Geometry check sheet. Reference: the model listing, model coordinates, mm. A direction names the side the tool comes from. Give positions to 0.01 mm unless a question says otherwise; leave off trailing zeros. Write each loop counter-clockwise with the first axis right and the second up, starting at its lowest first coordinate (ties: lowest second). Pieces come first, ordered by that corner, then holes. Notation, with made-up numbers: (-24, 79) -> (1, 79) arc R36 ccw to (1, 113) -> close; hole circle Ø2 at (58, -24.75). An arc over 180 degrees is marked (long way). Write item = value, one per line. Start each with the question number.
1. Depth check by flat-ended pin: P1, Ø4, axis at y = 3, z = -47, coming from the +X side; P2, Ø1, axis at x = -15.5, z = 21.5, coming from the -Y side; P3, Ø12, axis at x = 24, z = 34, coming from the +Y side. Enter the tip coordinate at first touch or a pass-through.
2. Cross-section at B-B, the plane x = -3.5. Record the cut outline in (y, z).
3. Mould release check, pull along X, two halves, no side actions. Record for faces 1 (the flat face through (34, -23.2, -20.9)), 2 (the cylindrical face through (-90.93, 39.923, -20.765)), 3 (the flat face through (10, -29, -70)): pulls with the +X half, pulls with the -X half, needs draft (parallel to the pull), parting line crosses it, or undercut.
4. Thickness scan on line 1 along Y through (x, z) = (37.7, 0); line 2 along Y through (x, z) = (35.45, 0); line 3 along X through (y, z) = (-13, -29). Record the ranges inside material, lowest first.
5. Set-up check for faces 4 (the flat face through (37.5, -12, -29)), 5 (the flat face through (-150, 1, -1)), 6 (the flat face through (47, 0, 0)), 7 (the cylindrical face through (-122.62, 37.18, -4.88)): record each of +Z, -Z, +X, -X, +Y, -Y from which the full face is reachable in a straight line by a thin tool's end or side.
6. Cross-section at A-A, the plane x = -120. Record the cut outline in (y, z), plus the area to 3 significant figures.
```python
from build123d import *

# Parameters (mm, degrees)
FILLET_1_R      = 5
FILLET_2_R      = 10
SKETCH_2_R      = 45
SKETCH_2_R_2    = 35
EXTRUDE_1_DEPTH = 32
SKETCH_3_R      = 35
EXTRUDE_2_DEPTH = 66
SKETCH_4_R      = 37.5
EXTRUDE_3_DEPTH = 54
SKETCH_5_R      = 45
EXTRUDE_4_DEPTH = 10
SKETCH_6_R      = 37.5
EXTRUDE_5_DEPTH = 54
SKETCH_9_R      = 31
EXTRUDE_8_DEPTH = 3.5
SKETCH_10_R     = 32.5
EXTRUDE_9_DEPTH = 9.5


with BuildPart() as part:
    # Sketch 1 → Revolve 1 (revolve)
    with BuildSketch(Plane.XY, mode=Mode.PRIVATE) as revolve_1_sk:
        Polygon((10, 100), (50, 100), (50, 55), (40, 55), (40, 35), (0, 35), (0, 70), (10, 70), align=None)
    revolve(revolve_1_sk.sketch.rotate(Axis((-1000, 0, 0), (1, 0, 0)), 90), axis=Axis((-1000, 0, 0), (1, 0, 0)))

    # Fillet 1
    fillet_1_edges = [part.edges().sort_by_distance(p)[0] for p in [
        (10, 0, -70),
        (50, 0, -100),
        (10, 0, -100),
    ]]
    fillet(fillet_1_edges, radius=FILLET_1_R)

    # Fillet 2
    fillet_2_edges = [part.edges().sort_by_distance(p)[0] for p in [
        (40, 0, -55),
    ]]
    fillet(fillet_2_edges, radius=FILLET_2_R - 0.0001)  # a hair under: the kernel refuses the full size



with BuildPart() as body_2:
    # Sketch 2 → Extrude 1 (new body)
    with BuildSketch(Plane.ZY):
        Circle(SKETCH_2_R)
        Circle(SKETCH_2_R_2, mode=Mode.SUBTRACT)
    extrude(amount=EXTRUDE_1_DEPTH)


with BuildPart() as part_1:
    add(part.part)

    add(body_2.part)  # Extrude 2 merges body 2
    # Sketch 3 → Extrude 2 (add)
    with BuildSketch(Plane.ZY.offset(32)):
        Circle(SKETCH_3_R)
    extrude(amount=-EXTRUDE_2_DEPTH)

    # Sketch 4 → Extrude 3 (add)
    with BuildSketch(Plane.ZY.offset(32)):
        Circle(SKETCH_4_R)
    extrude(amount=EXTRUDE_3_DEPTH)

    # Sketch 5 → Extrude 4 (add)
    with BuildSketch(Plane.ZY.offset(86)):
        with Locations(Location((0, 0, 0), (0, 0, 180))):
            Circle(SKETCH_5_R)
    extrude(amount=EXTRUDE_4_DEPTH)

    # Sketch 6 → Extrude 5 (add)
    with BuildSketch(Plane.ZY.offset(96)):
        Circle(SKETCH_6_R)
    extrude(amount=EXTRUDE_5_DEPTH)

    # Sketch 9 → Extrude 8 (add)
    with BuildSketch(Plane(origin=(34, 0, 0), x_dir=(0, 0, -1), z_dir=(1, 0, 0))):
        with Locations(Location((0, 0, 0), (0, 0, 180))):
            Circle(SKETCH_9_R)
    extrude(amount=EXTRUDE_8_DEPTH)

    # Sketch 10 → Extrude 9 (add)
    with BuildSketch(Plane(origin=(37.5, 0, 0), x_dir=(0, 0, -1), z_dir=(1, 0, 0))):
        Circle(SKETCH_10_R)
    extrude(amount=EXTRUDE_9_DEPTH)


solid = part_1.part
```
Answers:
q1.P1 = 40.88
q1.P2 = -39.8
q1.P3 = 96
q2.outline = circle Ø90 at (0, 0)
q3.face_1 = undercut
q3.face_2 = needs draft
q3.face_3 = pulls with the -X half
q4.line_1 = -100 to -35, -32.5 to 32.5, 35 to 100
q4.line_2 = -100 to -35, -31 to 31, 35 to 100
q4.line_3 = -150 to 34, 37.5 to 47
q5.face_4 = none
q5.face_5 = +Z, -Z, -X, +Y, -Y
q5.face_6 = +X
q5.face_7 = -X
q6.outline = circle Ø75 at (0, 0)
q6.area = 4,420 mm^2
